Check sheet for the modelled part. Datum: model origin and axes. Units: mm. A direction names the side the tool comes from. Round coordinates to 2 decimals unless told otherwise and drop trailing zeros. Loops run counter-clockwise (first coordinate to the right, second up) from the corner with the lowest first, then second, coordinate; pieces in that order, holes last. Notation, with made-up numbers: (-29, -5) - (-12, -5) arc R19 ccw to (-12, 9) - close; hole circle Ø10 at (9.25, -13). An arc over 180 degrees is marked (long way). Return JSON: item names as keys, results as strings.
Autodesk Inventor part; units mm, degrees
ref_plane "Work Plane1" through (0, 0, 2) normal (0, 0, 1) x (1, 0, 0)
ref_plane "Work Plane2" through (-11.127, 0, 0) normal (0, 1, 0) x (1, 0, 0)
ref_plane "YZ Plane" through (0, 0, 0) normal (1, 0, 0) x (0, 1, 0)
sketch "Sketch4" plane through (0, 0, 0) normal (0, 0, 1) x (1, 0, 0)
  line L0 (-20, -27.5) -> (20, -27.5)
  line L1 (20, -27.5) -> (20, 27.5)
  line L2 (20, 27.5) -> (-20, 27.5)
  line L3 (-20, 27.5) -> (-20, -27.5)
  line L4 (-20, -27.5) -> (20, 27.5) construction
  line L5 (20, -27.5) -> (-20, 27.5) construction
  circle A0 centre (0, 4) radius 1.5
  line L6 (-20, 27.5) -> (20, 27.5)
  line L7 (20, 27.5) -> (20, 23.5)
  line L8 (20, 23.5) -> (-20, 23.5)
  line L9 (-20, 23.5) -> (-20, 27.5)
  line L10 (-20, -27.5) -> (20, -27.5)
  line L11 (20, -27.5) -> (20, -23.5)
  line L12 (20, -23.5) -> (-20, -23.5)
  line L13 (-20, -23.5) -> (-20, -27.5)
  point P0 (0, 0)
  point P1 (-20, -23.5)
  dimension "d33" = 55
  dimension "d34" = 40
  dimension "d35" = 3
  dimension "d36" = 4
  dimension "d37" = 4
  dimension "d38" = 4
extrude "Extrusion4" add sketch "Sketch4" along normal blind 4 contours L3 L8 L1 L12
extrude "Extrusion5" add sketch "Sketch4" along normal blind 14 and the other way blind 10 contours L3 L12 L1 L0 | L3 L2 L1 L8
sketch "Sketch5" plane through (-20, -23.5, 4) normal (0, 1, 0) x (1, 0, 0)
  line L0 (0, 14) -> (0, -10)
  line L1 (0, 2) -> (40, 2)
  line L2 (40, 14) -> (40, -10)
  line L3 (5, -5.5) -> (35, -5.5)
  line L4 (35, -5.5) -> (35, 9.5)
  line L5 (35, 9.5) -> (5, 9.5)
  line L6 (5, 9.5) -> (5, -5.5)
  line L7 (5, -5.5) -> (35, 9.5) construction
  line L8 (35, -5.5) -> (5, 9.5) construction
  circle A0 centre (5, 9.5) radius 1.5
  circle A1 centre (35, 9.5) radius 1.5
  circle A2 centre (35, -5.5) radius 1.5
  circle A3 centre (5, -5.5) radius 1.5
  point P0 (20, 4)
  point P1 (20, 2)
  dimension "d45" = 15
  dimension "d46" = 30
  dimension "d47" = 3
  dimension "d48" = 3
  dimension "d49" = 3
  dimension "d50" = 3
extrude "Extrusion6" cut sketch "Sketch5" against normal blind 14 contours A0 L5 L6 | L6 L5 A0 | A3 L3 L6 | L6 L3 A3 | A2 L3 L4 | L4 L3 A2 | A1 L5 L4 | L4 L5 A1
sketch "Sketch6" plane through (-20, -23.5, 4) normal (0, 1, 0) x (1, 0, 0)
  circle A0 centre (5, -5.5) radius 1.5
  line L0 (5, -2.0359) -> (8, -3.7679)
  line L1 (8, -3.7679) -> (8, -7.2321)
  line L2 (8, -7.2321) -> (5, -8.9641)
  line L3 (5, -8.9641) -> (2, -7.2321)
  line L4 (2, -7.2321) -> (2, -3.7679)
  line L5 (2, -3.7679) -> (5, -2.0359)
  circle A1 centre (35, -5.5) radius 1.5
  line L6 (35, -8.9641) -> (32, -7.2321)
  line L7 (32, -7.2321) -> (32, -3.7679)
  line L8 (32, -3.7679) -> (35, -2.0359)
  line L9 (35, -2.0359) -> (38, -3.7679)
  line L10 (38, -3.7679) -> (38, -7.2321)
  line L11 (38, -7.2321) -> (35, -8.9641)
  circle A2 centre (5, -5.5) radius 1.5
  line L12 (40, -10) -> (0, -10)
  circle A3 centre (5, -5.5) radius 6.7268
  circle A4 centre (35, -5.5) radius 1.5
  line L13 (40, 14) -> (40, -10)
  circle A5 centre (35, -5.5) radius 6.7268
  circle A6 centre (35, -5.5) radius 1.5
  circle A7 centre (5, -5.5) radius 1.5
  line L14 (0, 0) -> (40, 0)
  line L15 (0, -10) -> (0, 0)
  line L16 (40, -10) -> (0, -10)
  line L17 (40, 0) -> (40, -10)
  point P0 (20, 4)
  point P1 (38.873, 0)
  point P2 (31.127, 0)
  point P3 (30, -10)
  point P4 (40, -1)
  point P5 (0, -1)
  point P6 (0, -10)
  point P7 (10, -10)
  point P8 (8.873, 0)
  point P9 (1.127, 0)
  dimension "d53" = 6
  dimension "d54" = 6
extrude "Extrusion7" add sketch "Sketch6" along normal blind 3.5 contours L12 A5 L14 L13 | A5 L14 L13 | L12 L15 A3 L14 | L15 L14 A3
ref_plane "Work Plane1" through (0, 0, 2) normal (0, 0, 1) x (1, 0, 0)
mirror "Mirror1" about plane through (0, 0, 2) normal (0, 0, 1) of "Extrusion7"
ref_plane "Work Plane2" through (-11.127, 0, 0) normal (0, 1, 0) x (1, 0, 0)
mirror "Mirror2" about plane through (-11.127, 0, 0) normal (0, 1, 0) of "Extrusion7", "Mirror1", "Extrusion6"
fillet "Fillet2" radius 5 4 edges at (-20, 23.75, 14) (-20, 23.75, -10) (20, 23.75, 14) (20, 23.75, -10)
fillet "Fillet3" radius 5 4 edges at (-20, -23.75, 14) (-20, -23.75, -10) (20, -23.75, 14) (20, -23.75, -10)
properties part number "DriverHolderInside"
Q1. Sectioned sample at C-C (x = -5.5). Enter the section's corners in (y, z), plus the area to 3 significant figures.
Answer key:
{"outline": "(-27.5, -10) - (-23.5, -10) - (-23.5, 0) - (23.5, 0) - (23.5, -10) - (27.5, -10) - (27.5, 14) - (23.5, 14) - (23.5, 4) - (-23.5, 4) - (-23.5, 14) - (-27.5, 14) - close", "area": "380 mm²"}
Q2. Sectioned sample at A-A (y = 4). Enter the section's corners in (x, z).
Answer key:
{"outline": "(-20, 0) - (-1.5, 0) - (-1.5, 4) - (-20, 4) - close; (1.5, 0) - (20, 0) - (20, 4) - (1.5, 4) - close"}
Q3. Draft check along X on faces 4 (the face through (-19, 24, 12)), 5 (the face through (20, 0, 2)), 6 (the face through (13.5, -25.47, -5.57)), 7 (the face through (0, 25, -10)). Enter one of: released by +X, released by -X, zero draft, split by the parting line, or undercut.
Answer key:
{"face 4": "released by -X", "face 5": "released by +X", "face 6": "undercut", "face 7": "zero draft"}
Q4. Tool access check on faces 1 (the face through (-13, -20, -3)), 2 (the face through (12, 22, 9)), 3 (the face through (-20, 0, 2)). Record the directions out of +Z, -Z, +X, -X, +Y, -Y that give a thin tool (end or side, any length) a straight path to the whole face; none if there is none.
Answer key:
{"face 1": "-Z, +X, -X", "face 2": "none", "face 3": "+Z, -Z, -X, +Y, -Y"}
Q5. Sectioned sample at B-B (x = 0). Enter the section's corners in (y, z).
Answer key:
{"outline": "(-27.5, -10) - (-23.5, -10) - (-23.5, 0) - (2.5, 0) - (2.5, 4) - (-23.5, 4) - (-23.5, 14) - (-27.5, 14) - close; (5.5, 0) - (23.5, 0) - (23.5, -10) - (27.5, -10) - (27.5, 14) - (23.5, 14) - (23.5, 4) - (5.5, 4) - close"}
Q6. Depth check by flat-ended pin: P1, Ø12, axis at x = 4.5, y = 7, coming from the -Z side; P2, Ø3, axis at y = 22, z = -6, coming from the +X side; P3, Ø3, axis at x = -13, y = -15.5, coming from the +Z side; P4, Ø1.7, axis at y = 21, z = -6, coming from the -X side. Enter the tip coordinate at first touch or a pass-through.
Answer key:
{"P1": "stops at z = 0", "P2": "stops at x = 20", "P3": "stops at z = 4", "P4": "stops at x = -20"}
Q7. Sectioned sample at D-D (y = -15). Enter the section's corners in (x, z).
Answer key:
{"outline": "(-20, 0) - (20, 0) - (20, 4) - (-20, 4) - close"}
Q8. Scan lines: probe 1 along Z at (x, y) = (-15, -25); probe 2 along Y at (x, z) = (14.5, 4.5); probe 3 along Y at (x, z) = (-6, 11.75). Record each from-to range of solid material in increasing order. Write a range as [from, to].
Answer key:
{"probe 1": "z = [-10, -7], [-4, 8], [11, 14]", "probe 2": "y = [-27.5, -20], [20, 27.5]", "probe 3": "y = [-27.5, -23.5], [23.5, 27.5]"}
